Can you work these out from the model? Positions are in its coordinate system, mm. Coordinates: 2 decimals unless noted, no trailing zeros. Write each loop counter-clockwise with the first axis right and the second up, starting at its lowest first coordinate (ties: lowest second). Pieces come first, ordered by that corner, then holes. Notation, with made-up numbers: (44, 44) -> (80, 44) arc R26 ccw to (80, 60) -> close; hole circle Ø1 at (8, -18). An arc over 180 degrees is marked (long way). Answer as CSV lines item,"result". Start each with the question number.
```python
from build123d import *

# Parameters (mm, degrees)
SKETCH1_R           = 11.43
SKETCH1_R_2         = 2.38125
BOSS_EXTRUDE1_DEPTH = 4.7625


with BuildPart() as part:
    # Sketch1 → Boss-Extrude1 (new body)
    with BuildSketch(Plane.XY):
        with BuildLine():
            Line((-28.575, 19.05), (10.795, 19.05))
            ThreePointArc((10.795, 19.05), (23.367358569, 13.842358569), (28.575, 1.27))
            Line((28.575, 1.27), (28.575, -1.27))
            ThreePointArc((28.575, -1.27), (23.367358569, -13.842358569), (10.795, -19.05))
            Line((10.795, -19.05), (-28.575, -19.05))
            Line((-28.575, -19.05), (-28.575, 19.05))
        make_face()
        with Locations(Location((14.605, 0, 0), (0, 0, 180))):
            Circle(SKETCH1_R, mode=Mode.SUBTRACT)
        with Locations(Location((-15.875, 12.7, 0), (0, 0, 180))):
            Circle(SKETCH1_R_2, mode=Mode.SUBTRACT)
        with Locations(Location((-15.875, -12.7, 0), (0, 0, 180))):
            Circle(SKETCH1_R_2, mode=Mode.SUBTRACT)
    extrude(amount=BOSS_EXTRUDE1_DEPTH)


solid = part.part
```
Q1. For pin 1 (4.5 mm diameter, centred on x = -15.875, y = 12.7, fed in from -Z), with a flat end and sliding along its axis, tell me the tip position at first contact or that it passes through.
Q2. Imagine slicing it at C-C (x = 15). Write out the boundary of the cut face in (y, z).
Q3. Imagine slicing it at B-B (y = 0). Write out the boundary of the cut face in (x, z) (1 decimal), then the cut area to 3 significant figures.
Q4. Imagine slicing it at A-A (z = 1.45). State how many separate pieces and enclosed holes the cut face has, then the cut area to 3 significant figures.
Q5. If we mould it in two halves opening along X, with no side actions, what happens to faces 1 (the face through (-9, -19.05, 2)), 2 (the face through (23.23, 13.98, 2.35)), 3 (the face through (-28.575, 0, 2)), 4 (the face through (3.7, -3.43, 2.35))? For each: released by +X, released by -X, zero draft, split by the parting line, or undercut.
Q6. I need wall thicknesses on L1, parallel to Y at x = -15, z = 0.5; L2, parallel to X at y = 12.7, z = 3.25 (3 decimals); L3, parallel to Y at x = 8.5, z = 4.05. Which ranges of each line are inside material? Lowest first, please.
Entries:
1,pin 1,"through"
2,outline,"(-18.55, 0) -> (-11.42, 0) -> (-11.42, 4.76) -> (-18.55, 4.76) -> close; (11.42, 0) -> (18.55, 0) -> (18.55, 4.76) -> (11.42, 4.76) -> close"
3,outline,"(-28.6, 0) -> (3.2, 0) -> (3.2, 4.8) -> (-28.6, 4.8) -> close; (26, 0) -> (28.6, 0) -> (28.6, 4.8) -> (26, 4.8) -> close"
3,area,"163 mm2"
4,separate pieces,"1"
4,enclosed holes,"3"
4,area,"1,600 mm2"
5,face 1,"zero draft"
5,face 2,"released by +X"
5,face 3,"released by -X"
5,face 4,"undercut"
6,L1,"-19.05 to -14.91, -10.49 to 10.49, 14.91 to 19.05"
6,L2,"-28.575 to -18.256, -13.494 to 24.414"
6,L3,"-19.05 to -9.66, 9.66 to 19.05"
